Here's how the part is built. I have some questions about the finished solid (model axes, mm). Face numbers are marked on the shaded views. A direction names the side the tool comes from. Give positions to 0.01 mm unless a question says otherwise; leave off trailing zeros. Loops run counter-clockwise (first coordinate to the right, second up) from the corner with the lowest first, then second, coordinate; pieces in that order, holes last.
Q1. We'd pull the mould along Z, two halves only. Please class the marked faces 5, 6 and 7: +Z half, -Z half, draft (parallel to the pull), parting line (faces both ways), or undercut.
Q2. If we section it at C-C (y = -5): Please give me the cut outline in (x, z), plus the area to 3 significant figures.
Q3. If we section it at A-A (x = -14): Please give me the cut outline in (y, z), plus the area to 3 significant figures.
Q4. I need wall thicknesses on line 1 (X direction, y = 5, z = 9); line 2 (Z direction, x = -28, y = 10); line 3 (X direction, y = -16, z = 6). Which ranges of each line are inside material? Lowest first, please.
Q5. Will these pins go through, and if not, where does the flat tip stop? P1, Ø0.5, axis at x = 1, y = -20, coming from the +Z side; P2, Ø5, axis at x = -24.5, z = 11, coming from the -Y side; P3, Ø5, axis at x = 3, z = 16, coming from the +Y side.
Q6. If we section it at B-B (z = 8): Please give me the cut outline in (x, y).
Q7. If we section it at D-D (x = -6): Please give me the cut outline in (y, z).
Q8. For the marked faces 1, 2, 3 and 4, which set-ups out of +Z, -Z, +X, -X, +Y, -Y let a thin tool reach every point of the face, with its end or its side?
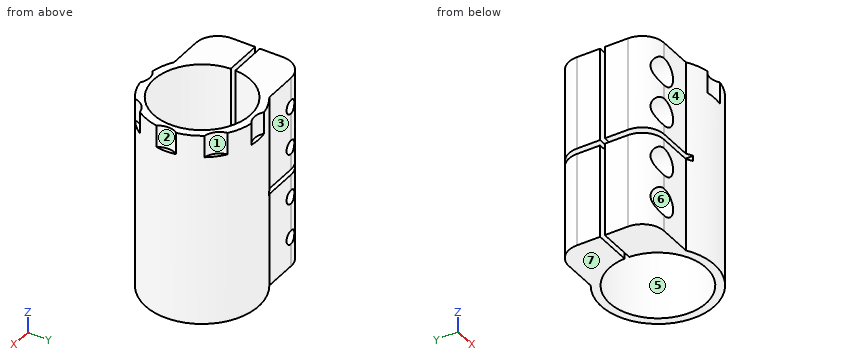
from build123d import *

# Parameters (mm, degrees)
F1_DEPTH       = 35
F3_D           = 5
F3_START       = 1.7550021
F3_CBORE_D     = 10
F3_CBORE_DEPTH = 8
F4_W           = 22.4
F4_H           = 2
F5_DEPTH       = 350
F7_DEPTH       = 8


with BuildPart() as f1:
    # F0 (on Top) → F1 (new body, symmetric)
    with BuildSketch(Plane.XY):
        with BuildLine():
            ThreePointArc((-17.4795348609, 0.84608572), (17.5, 0), (-17.4795348609, -0.84608572))
            Line((-17.4795348609, -0.84608572), (-20.4825325327, -0.84608572))
            Line((-20.4825325327, -0.84608572), (-31.2825325327, -0.84608572))
            Line((-31.2825325327, -0.84608572), (-31.2825325327, -9.24608572))
            ThreePointArc((-31.2825325327, -9.24608572), (-28.9393867822, -14.9029399695), (-23.2825325327, -17.24608572))
            Line((-23.2825325327, -17.24608572), (-11.0825325327, -17.24608572))
            ThreePointArc((-11.0825325327, -17.24608572), (20.5, 0), (-11.0825325327, 17.24608572))
            Line((-11.0825325327, 17.24608572), (-23.2825325327, 17.24608572))
            ThreePointArc((-23.2825325327, 17.24608572), (-28.9393867822, 14.9029399695), (-31.2825325327, 9.24608572))
            Line((-31.2825325327, 9.24608572), (-31.2825325327, 0.84608572))
            Line((-31.2825325327, 0.84608572), (-20.4825325327, 0.84608572))
            Line((-20.4825325327, 0.84608572), (-17.4795348609, 0.84608572))
        make_face()
    extrude(amount=F1_DEPTH, both=True)

    # F3 (through all)
    # its depths count from where the whole tool has entered the part; down to there all is cleared
    with Locations(Plane.XZ.offset(17.24608572).offset(-F3_START)):
        with Locations((-23.2825325327, -24.25), (-23.2825325327, -9.25), (-23.2825325327, 9.25), (-23.2825325327, 24.25)):
            CounterBoreHole(F3_D / 2, F3_CBORE_D / 2, F3_CBORE_DEPTH)

    # F4 (on face) → F5 (cut, symmetric)
    with BuildSketch(Plane.XZ.offset(17.24608572)):
        with Locations((-20.0825325327, 0)):
            Rectangle(F4_W, F4_H)
    extrude(amount=F5_DEPTH, both=True, mode=Mode.SUBTRACT)

    # F6 (on face) → F7 (cut)
    with BuildSketch(Plane.XY.offset(35)):
        with BuildLine():
            ThreePointArc((-3.5799127084, -20.185), (0, -20.5), (3.5799127084, -20.185))
            ThreePointArc((3.5799127084, -20.185), (0, -19), (-3.5799127084, -20.185))
        make_face()
        with BuildLine():
            ThreePointArc((16.8043309304, -11.7415698261), (13.4350288425, -13.4350288425), (11.7415698261, -16.8043309304))
            ThreePointArc((11.7415698261, -16.8043309304), (14.4956890143, -14.4956890143), (16.8043309304, -11.7415698261))
        make_face()
        with BuildLine():
            ThreePointArc((20.185, 3.5799127084), (19, 0), (20.185, -3.5799127084))
            ThreePointArc((20.185, -3.5799127084), (20.5, 0), (20.185, 3.5799127084))
        make_face()
        with BuildLine():
            ThreePointArc((11.7415698261, 16.8043309304), (13.4350288425, 13.4350288425), (16.8043309304, 11.7415698261))
            ThreePointArc((16.8043309304, 11.7415698261), (14.4956890143, 14.4956890143), (11.7415698261, 16.8043309304))
        make_face()
        with BuildLine():
            ThreePointArc((-3.5799127084, 20.185), (0, 19), (3.5799127084, 20.185))
            ThreePointArc((3.5799127084, 20.185), (0, 20.5), (-3.5799127084, 20.185))
        make_face()
    extrude(amount=-F7_DEPTH, mode=Mode.SUBTRACT)


solid = f1.part
Check sheet entries:
1. face 5: draft
1. face 6: undercut
1. face 7: -Z half
2. outline: (-31.28, -35) - (-16.77, -35) - (-16.77, -1) - (-31.28, -1) - close; (-31.28, 1) - (-16.77, 1) - (-16.77, 35) - (-31.28, 35) - close; (16.77, -35) - (19.88, -35) - (19.88, 35) - (16.77, 35) - close; hole circle Ø5 at (-23.28, -24.25); hole circle Ø5 at (-23.28, -9.25); hole circle Ø5 at (-23.28, 9.25); hole circle Ø5 at (-23.28, 24.25)
2. area: 1,130 mm2
3. outline: (-17.25, -35) - (-10.5, -35) - (-10.5, -1) - (-17.25, -1) - close; (-17.25, 1) - (-10.5, 1) - (-10.5, 35) - (-17.25, 35) - close; (10.5, -35) - (17.25, -35) - (17.25, -1) - (10.5, -1) - close; (10.5, 1) - (17.25, 1) - (17.25, 35) - (10.5, 35) - close
3. area: 917 mm2
4. line 1: x = -31.28 to -25.77, -20.8 to -16.77, 16.77 to 19.88
4. line 2: z = -35 to -1, 1 to 35
4. line 3: x = -27.57 to -27.08, -19.48 to -7.09, 7.09 to 12.82
5. P1: stops at z = 27
5. P2: stops at y = -7.49
5. P3: stops at y = 20.49
6. outline: (-31.28, -9.25) arc R8 ccw to (-28.12, -15.61) - (-28.12, -7.49) - (-25.45, -7.49) - (-25.45, -0.85) - (-31.28, -0.85) - close; (-31.28, 0.85) - (-25.45, 0.85) - (-25.45, 16.95) arc R8 ccw to (-31.28, 9.25) - close; (-21.12, -7.49) - (-18.44, -7.49) - (-18.44, -17.25) - (-11.08, -17.25) arc R20.5 ccw (long way) to (-11.08, 17.25) - (-21.12, 17.25) - (-21.12, 0.85) - (-17.48, 0.85) arc R17.5 cw (long way) to (-17.48, -0.85) - (-21.12, -0.85) - close
7. outline: (-19.6, -35) - (-16.44, -35) - (-16.44, 35) - (-19.6, 35) - close; (16.44, -35) - (19.6, -35) - (19.6, 35) - (16.44, 35) - close
8. face 1: +Z, +X, +Y
8. face 2: +Z, +X
8. face 3: +Z, -Z, -X, +Y
8. face 4: +Z, -Z, -X, -Y
